```python
from build123d import *

# Parameters (mm, degrees)
SKETCH1_W                                            = 50
SKETCH1_H                                            = 70
SKETCH1_R                                            = 1.35
SKETCH1_R_2                                          = 1.5
BOSS_EXTRUDE1_DEPTH                                  = 7
CHAMFER1_SIZE                                        = 2
CHAMFER2_SIZE                                        = 2
CHAMFER3_SIZE                                        = 2
CHAMFER4_SIZE                                        = 2
CSK_FOR_M4_COUNTERSUNK_FLAT_HEAD_SCREW1_D            = 4.5
CSK_FOR_M4_COUNTERSUNK_FLAT_HEAD_SCREW1_DEPTH        = 7
CSK_FOR_M4_COUNTERSUNK_FLAT_HEAD_SCREW1_CSINK_D      = 9.4
CSK_FOR_M4_COUNTERSUNK_FLAT_HEAD_SCREW1_CSINK_ANGLE  = 90
CBORE_FOR_M2_5_HEX_SOCKET_HEAD_CAP_SCREW_D           = 2.9
CBORE_FOR_M2_5_HEX_SOCKET_HEAD_CAP_SCREW_CBORE_D     = 5.5
CBORE_FOR_M2_5_HEX_SOCKET_HEAD_CAP_SCREW_CBORE_DEPTH = 2.9


with BuildPart() as part:
    # Sketch1 → Boss-Extrude1 (new body)
    with BuildSketch(Plane.XY):
        Rectangle(SKETCH1_W, SKETCH1_H)
        with Locations(Location((11, 20, 0), (0, 0, 180))):
            Circle(SKETCH1_R, mode=Mode.SUBTRACT)
        with Locations(Location((-11, 20, 0), (0, 0, 180))):
            Circle(SKETCH1_R, mode=Mode.SUBTRACT)
        with Locations(Location((-11, -20, 0), (0, 0, 180))):
            Circle(SKETCH1_R, mode=Mode.SUBTRACT)
        with Locations(Location((11, -20, 0), (0, 0, 180))):
            Circle(SKETCH1_R, mode=Mode.SUBTRACT)
        with Locations(Location((18, 28.5, 0), (0, 0, 180))):
            Circle(SKETCH1_R_2, mode=Mode.SUBTRACT)
        with Locations(Location((-18, 28.5, 0), (0, 0, 180))):
            Circle(SKETCH1_R_2, mode=Mode.SUBTRACT)
        with Locations(Location((-18, -28.5, 0), (0, 0, 180))):
            Circle(SKETCH1_R_2, mode=Mode.SUBTRACT)
        with Locations(Location((18, -28.5, 0), (0, 0, 180))):
            Circle(SKETCH1_R_2, mode=Mode.SUBTRACT)
    extrude(amount=BOSS_EXTRUDE1_DEPTH)

    # Chamfer1
    chamfer1_edges = [part.edges().sort_by_distance(p)[0] for p in [
        (-25, 35, 3.5),
    ]]
    chamfer(chamfer1_edges, length=CHAMFER1_SIZE)

    # Chamfer2
    chamfer2_edges = [part.edges().sort_by_distance(p)[0] for p in [
        (-25, -35, 3.5),
    ]]
    chamfer(chamfer2_edges, length=CHAMFER2_SIZE)

    # Chamfer3
    chamfer3_edges = [part.edges().sort_by_distance(p)[0] for p in [
        (25, -35, 3.5),
    ]]
    chamfer(chamfer3_edges, length=CHAMFER3_SIZE)

    # Chamfer4
    chamfer4_edges = [part.edges().sort_by_distance(p)[0] for p in [
        (25, 35, 3.5),
    ]]
    chamfer(chamfer4_edges, length=CHAMFER4_SIZE)

    # CSK for M4 Countersunk Flat Head Screw1
    with Locations(Plane.XY.offset(7)):
        with Locations((18, 28.5), (18, -28.5), (-18, -28.5), (-18, 28.5)):
            CounterSinkHole(CSK_FOR_M4_COUNTERSUNK_FLAT_HEAD_SCREW1_D / 2, CSK_FOR_M4_COUNTERSUNK_FLAT_HEAD_SCREW1_CSINK_D / 2, depth=CSK_FOR_M4_COUNTERSUNK_FLAT_HEAD_SCREW1_DEPTH, counter_sink_angle=CSK_FOR_M4_COUNTERSUNK_FLAT_HEAD_SCREW1_CSINK_ANGLE)

    # CBORE for M2.5 Hex Socket Head Cap Screw1 (through all)
    with Locations(Plane(origin=(0, 0, 0), x_dir=(-1, 0, 0), z_dir=(0, 0, -1))):
        with Locations((11, 20), (-11, 20), (-11, -20), (11, -20)):
            CounterBoreHole(CBORE_FOR_M2_5_HEX_SOCKET_HEAD_CAP_SCREW_D / 2, CBORE_FOR_M2_5_HEX_SOCKET_HEAD_CAP_SCREW_CBORE_D / 2, CBORE_FOR_M2_5_HEX_SOCKET_HEAD_CAP_SCREW_CBORE_DEPTH)


solid = part.part
```
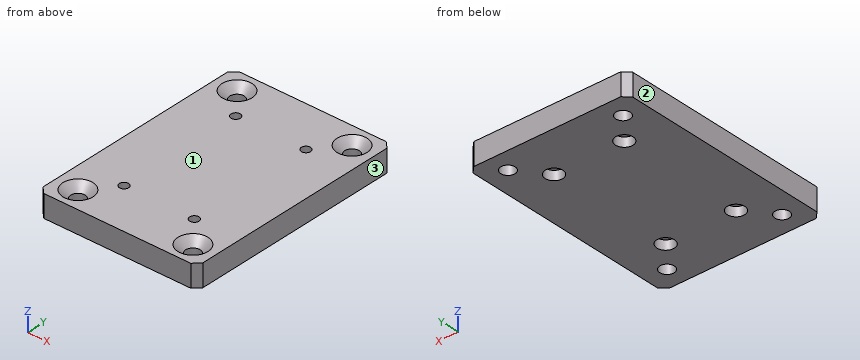
Geometry check sheet. Reference: the model listing, model coordinates, mm. Face numbers are marked on the shaded views. Give positions to 0.01 mm unless a question says otherwise; leave off trailing zeros. Write each loop counter-clockwise with the first axis right and the second up, starting at its lowest first coordinate (ties: lowest second). Pieces come first, ordered by that corner, then holes.
1) Section check C-C, the plane y = -28.5. Record the boundary of the cut face in (x, z).
2) Gauge pin test, flat ends, axial feed: pin 1 (7 mm diameter, centred on x = -18, y = 28.5, fed in from +Z); pin 2 (5 mm diameter, centred on x = -18, y = -28.5, fed in from +Z); pin 3 (1.6 mm diameter, centred on x = -10.5, y = 21, fed in from -Z). Record the tip position at first contact, or that the pin passes through.
3) Release check for a two-part mould opening along X. For the marked faces 1, 2 and 3 record: pulls with the +X half, pulls with the -X half, needs draft (parallel to the pull), parting line crosses it, or undercut.
4) Section check A-A, the plane y = 20. Record the boundary of the cut face in (x, z).
5) Material ranges on L1, parallel to Y at x = 11, z = 5.35; L2, parallel to X at y = 28.5, z = 3.35; L3, parallel to Y at x = -18, z = 1.5, recorded low to high.
6) Section check B-B, the plane z = 2. State how many separate pieces and enclosed holes the cut face has, and give its area (3 significant figures).
Computed:
1. outline: (-25, 0) - (-20.25, 0) - (-20.25, 4.55) - (-22.7, 7) - (-25, 7) - close; (-15.75, 0) - (15.75, 0) - (15.75, 4.55) - (13.3, 7) - (-13.3, 7) - (-15.75, 4.55) - close; (20.25, 0) - (25, 0) - (25, 7) - (22.7, 7) - (20.25, 4.55) - close
2. pin 1: stops at z = 5.8
2. pin 2: stops at z = 4.8
2. pin 3: stops at z = 2.9
3. face 1: needs draft
3. face 2: pulls with the -X half
3. face 3: pulls with the +X half
4. outline: (-25, 0) - (-13.75, 0) - (-13.75, 2.9) - (-12.45, 2.9) - (-12.45, 7) - (-25, 7) - close; (-9.55, 2.9) - (-8.25, 2.9) - (-8.25, 0) - (8.25, 0) - (8.25, 2.9) - (9.55, 2.9) - (9.55, 7) - (-9.55, 7) - close; (12.45, 2.9) - (13.75, 2.9) - (13.75, 0) - (25, 0) - (25, 7) - (12.45, 7) - close
5. L1: y = -35 to -21.45, -18.55 to 18.55, 21.45 to 35
5. L2: x = -25 to -20.25, -15.75 to 15.75, 20.25 to 25
5. L3: y = -35 to -30.75, -26.25 to 26.25, 30.75 to 35
6. separate pieces: 1
6. enclosed holes: 8
6. area: 3,330 mm2
